```python
from build123d import *
from build123d.topology import SkipClean

# Parameters (mm, degrees)
SKETCH2_R            = 1.55
SKETCH2_R_2          = 15.6
BOSS_EXTRUDE1_DEPTH  = 5
BOSS_EXTRUDE3_DEPTH  = 41
BOSS_EXTRUDE4_DEPTH  = 7.5
BOSS_EXTRUDE5_DEPTH  = 3
BOSS_EXTRUDE6_START  = -7.5
BOSS_EXTRUDE6_DEPTH  = 10.5
SKETCH12_W           = 10.5
SKETCH12_H           = 5
BOSS_EXTRUDE8_DEPTH  = 23.65
SKETCH13_W           = 10.5
SKETCH13_H           = 5
BOSS_EXTRUDE9_DEPTH  = 23.65
SKETCH14_W           = 5
SKETCH14_H           = 28.65
CUT_EXTRUDE1_DEPTH   = 41
SKETCH15_W           = 5
SKETCH15_H           = 10.5
BOSS_EXTRUDE10_DEPTH = 13.449158782
BOSS_EXTRUDE11_DEPTH = 5
BOSS_EXTRUDE12_DEPTH = 5


# Read off the part's stored shape, not the designer's step: Boss-Extrude6
with BuildPart() as part:
    # Sketch2 → Boss-Extrude1 (new body)
    with BuildSketch(Plane.XY):
        Polygon((-10.909227683, 21.454823411), (23.390772317, 21.454823411), (27.390772317, 17.454823411), (27.390772317, -16.845176589), (23.390772317, -20.845176589), (-10.909227683, -20.845176589), (-14.909227683, -16.845176589), (-14.909227683, 17.454823411), align=None)
        with Locations((-9.359227683, 15.904823411)):
            Circle(SKETCH2_R, mode=Mode.SUBTRACT)
        with Locations(Location((21.840772317, 15.904823411, 0), (0, 0, 180))):
            Circle(SKETCH2_R, mode=Mode.SUBTRACT)
        with Locations((21.840772317, -15.295176589)):
            Circle(SKETCH2_R, mode=Mode.SUBTRACT)
        with Locations(Location((-9.359227683, -15.295176589, 0), (0, 0, 180))):
            Circle(SKETCH2_R, mode=Mode.SUBTRACT)
        with Locations((6.240772317, 0.304823411)):
            Circle(SKETCH2_R_2, mode=Mode.SUBTRACT)
    extrude(amount=BOSS_EXTRUDE1_DEPTH)

    # Sketch4 → Boss-Extrude3 (add)
    with BuildSketch(Plane.XY.offset(5)):
        Polygon((-14.909227683, -12.195176589), (-14.909227683, 0.304823411), (-14.909227683, 12.804823411), (-19.909227683, 12.804823411), (-19.909227683, -12.195176589), (-19.909227683, -20.951034478), (-10.909227683, -20.845176589), (-14.909227683, -16.845176589), align=None)
        Polygon((32.390772317, 12.804823411), (27.390772317, 12.804823411), (27.390772317, 0.304823411), (27.390772317, -12.195176589), (27.390772317, -16.845176589), (23.390772317, -20.845176589), (32.390772317, -21.056892366), (32.390772317, -12.195176589), align=None)
    extrude(amount=-BOSS_EXTRUDE3_DEPTH)

    # Sketch12 → Boss-Extrude8 (add)
    with BuildSketch(Plane.ZY.offset(-3.740772317)):
        with Locations((-41.25, -18.345176589)):
            Rectangle(SKETCH12_W, SKETCH12_H)
    extrude(amount=BOSS_EXTRUDE8_DEPTH)

    # Sketch13 → Boss-Extrude9 (add)
    with BuildSketch(Plane(origin=(8.740772317, 0, 0), x_dir=(0, 0, -1), z_dir=(1, 0, 0))):
        with Locations((41.25, -18.345176589)):
            Rectangle(SKETCH13_W, SKETCH13_H)
    extrude(amount=BOSS_EXTRUDE9_DEPTH)

    # Sketch14 → Cut-Extrude1 (cut)
    with BuildSketch(Plane(origin=(0, 0, -36), x_dir=(-1, 0, 0), z_dir=(0, 0, -1))):
        with Locations((-29.890772317, -1.520176589)):
            Rectangle(SKETCH14_W, SKETCH14_H)
        with Locations((17.409227683, -1.520176589)):
            Rectangle(SKETCH14_W, SKETCH14_H)
    extrude(amount=-CUT_EXTRUDE1_DEPTH, mode=Mode.SUBTRACT)



with BuildPart() as body_2:
    # Sketch5 → Boss-Extrude4 (new body)
    with BuildSketch(Plane(origin=(0, 0, -36), x_dir=(-1, 0, 0), z_dir=(0, 0, -1))):
        with BuildLine():
            ThreePointArc((1.459227683, 4.190775675), (-6.240772317, -8.320176589), (-13.940772317, 4.190775675))
            Line((-13.940772317, 4.190775675), (-13.940772317, 11.190775675))
            Line((-13.940772317, 11.190775675), (-13.940772317, 14.190775675))
            Line((-13.940772317, 14.190775675), (-16.940772317, 14.190775675))
            Line((-16.940772317, 14.190775675), (-16.940772317, 4.849119286))
            ThreePointArc((-16.940772317, 4.849119286), (-6.240772317, -11.320176589), (4.459227683, 4.849119286))
            Line((4.459227683, 4.849119286), (4.459227683, 14.190775675))
            Line((4.459227683, 14.190775675), (1.459227683, 14.190775675))
            Line((1.459227683, 14.190775675), (1.459227683, 11.190775675))
            Line((1.459227683, 11.190775675), (1.459227683, 4.190775675))
        make_face()
    extrude(amount=BOSS_EXTRUDE4_DEPTH)

    # Sketch6 → Boss-Extrude5 (add)
    with SkipClean():  # the faces are left unmerged after this step: merging them gives an invalid solid
        with BuildSketch(Plane(origin=(0, 0, -43.5), x_dir=(-1, 0, 0), z_dir=(0, 0, -1))):
            with BuildLine():
                Line((-16.940772317, 4.849119286), (-16.940772317, 14.190775675))
                Line((-16.940772317, 14.190775675), (4.459227683, 14.190775675))
                Line((4.459227683, 14.190775675), (4.459227683, 4.849119286))
                ThreePointArc((4.459227683, 4.849119286), (-6.240772317, -11.320176589), (-16.940772317, 4.849119286))
            make_face()
        extrude(amount=BOSS_EXTRUDE5_DEPTH)

    # Boss-Extrude6 outline → Boss-Extrude6 (add)
    with SkipClean():  # the faces are left unmerged after this step: merging them gives an invalid solid
        with BuildSketch(Plane(origin=(0, 0, -43.5), x_dir=(-1, 0, 0), z_dir=(0, 0, -1)).offset(BOSS_EXTRUDE6_START)):
            with BuildLine():
                Line((-8.740772317, -20.845176589), (-3.740772317, -20.845176589))
                Line((-3.740772317, -20.845176589), (-3.740772317, -11.048177294))
                ThreePointArc((-3.740772317, -11.048177294), (-6.240772317, -11.320176589), (-8.740772317, -11.048177294))
                Line((-8.740772317, -11.048177294), (-8.740772317, -20.845176589))
            make_face()
            with BuildLine():
                Line((-32.390772317, -2.396017807), (-17.547676478, -2.396017807))
                ThreePointArc((-17.547676478, -2.396017807), (-17.863953086, 0.099168806), (-17.636143917, 2.603982193))
                Line((-17.636143917, 2.603982193), (-32.390772317, 2.603982193))
                Line((-32.390772317, 2.603982193), (-32.390772317, -2.396017807))
            make_face()
            with BuildLine():
                ThreePointArc((5.154599283, 2.603982193), (5.382408452, 0.099168806), (5.066131844, -2.396017807))
                Line((5.066131844, -2.396017807), (19.909227683, -2.396017807))
                Line((19.909227683, -2.396017807), (19.909227683, 2.603982193))
                Line((19.909227683, 2.603982193), (5.154599283, 2.603982193))
            make_face()
        extrude(amount=BOSS_EXTRUDE6_DEPTH)


with BuildPart() as part_1:
    with SkipClean():  # the faces are left unmerged after this step: merging them gives an invalid solid
        add(part.part)

        add(body_2.part)  # Boss-Extrude10 merges body 2
        # Sketch15 → Boss-Extrude10 (add)
        with BuildSketch(Plane(origin=(0, -15.845176589, 0), x_dir=(1, 0, 0), z_dir=(0, 1, 0))):
            with Locations((29.890772317, 41.25)):
                Rectangle(SKETCH15_W, SKETCH15_H)
            with Locations((-17.409227683, 41.25)):
                Rectangle(SKETCH15_W, SKETCH15_H)
        extrude(amount=BOSS_EXTRUDE10_DEPTH)

    # Sketch16 → Boss-Extrude11 (add)
    with SkipClean():  # the faces are left unmerged after this step: merging them gives an invalid solid
        with BuildSketch(Plane(origin=(32.390772317, 0, 0), x_dir=(0, 0, -1), z_dir=(1, 0, 0))):
            Polygon((36, -10.845176589), (31, -15.845176589), (36, -15.845176589), align=None)
        extrude(amount=-BOSS_EXTRUDE11_DEPTH)

    # Sketch18 → Boss-Extrude12 (add)
    with SkipClean():  # the faces are left unmerged after this step: merging them gives an invalid solid
        with BuildSketch(Plane.ZY.offset(19.909227683)):
            Polygon((-36, -10.845176589), (-31, -15.845176589), (-36, -15.845176589), align=None)
        extrude(amount=-BOSS_EXTRUDE12_DEPTH)


solid = part_1.part
```
Verification items for the finished model (mm, model axes). A direction names the side the tool comes from. Give positions to 0.01 mm unless a question says otherwise; leave off trailing zeros. Order: outer loops, then holes, each group sorted by start corner. A loop starts at its lowest first (then second) coordinate and runs counter-clockwise, first axis right, second up. Notation, with made-up numbers: (55, 86.5) - (74, 86.5) arc R15 cw to (74, 109.5) - close; hole circle Ø7 at (11, -38.75). An arc over 180 degrees is marked (long way). Answer as CSV lines item,"result". Start each with the question number.
Item 1: Section check C-C, the plane z = -42. Record the boundary of the cut face in (x, y) (3 decimals), plus the area to 3 significant figures.
Item 2: Section check A-A, the plane z = -3. Record the boundary of the cut face in (x, y).
Item 3: Section check D-D, the plane y = -6. Record the boundary of the cut face in (x, z).
Item 4: Gauge pin test, flat ends, axial feed: pin 1 (6 mm diameter, centred on y = 10.5, z = -39.5, fed in from +X); pin 2 (3 mm diameter, centred on x = -10, z = -39, fed in from -Y); pin 3 (10 mm diameter, centred on y = -11.5, z = -32.5, fed in from +X); pin 4 (6 mm diameter, centred on y = 7.5, z = -39, fed in from -X). Record the tip position at first contact, or that the pin passes through.
Item 5: Mould release check, pull along X, two halves, no side actions. Record for faces 1 (the face through (29.926, -13.31, -33.535)), 2 (the face through (27.391, 1, 2)), 3 (the face through (6, -20.845, 2)): released by +X, released by -X, zero draft, split by the parting line, or undercut.
Item 6: Material ranges on L1, parallel to X at y = -13, z = -42.5; L2, parallel to Z at x = 11, y = 4; L3, parallel to Y at x = 28.5, z = -17, recorded low to high.
Item 7: Access from +Z, -Z, +X, -X, +Y, -Y to the whole of each face (thin tool, end or side, straight path). Record for faces 4 (the face through (-3, 15, 0)), 5 (the face through (-10, -2.396, -41)), 6 (the face through (22.674, -13.988, 2.465)).
Filled in:
1,outline,"(-19.909, -20.845) - (32.391, -20.845) - (32.391, 2.604) - (17.636, 2.604) arc R11.625 ccw to (16.941, 4.849) - (16.941, 14.191) - (13.941, 14.191) - (13.941, 4.191) arc R8.625 cw (long way) to (-1.459, 4.191) - (-1.459, 14.191) - (-4.459, 14.191) - (-4.459, 4.849) arc R11.625 ccw to (-5.155, 2.604) - (-19.909, 2.604) - close; hole (-14.909, -15.845) - (3.741, -15.845) - (3.741, -11.048) arc R11.625 cw to (-5.066, -2.396) - (-14.909, -2.396) - close; hole (8.741, -15.845) - (27.391, -15.845) - (27.391, -2.396) - (17.548, -2.396) arc R11.625 cw to (8.741, -11.048) - close"
1,area,"745 mm^2"
2,outline,"(-19.91, -20.95) - (-10.91, -20.85) - (-14.91, -16.85) - (-14.91, -15.85) - (-19.91, -15.85) - close; (23.39, -20.85) - (32.39, -21.06) - (32.39, -15.85) - (27.39, -15.85) - (27.39, -16.85) - close"
3,outline,"(-19.91, -46.5) - (-14.91, -46.5) - (-14.91, -36) - (-19.91, -36) - close; (-14.91, 0) - (-8.03, 0) - (-8.03, 5) - (-14.91, 5) - close; (-3.53, -46.5) - (16.01, -46.5) - (16.01, -36) - (12.13, -36) - (12.13, -43.5) - (0.36, -43.5) - (0.36, -36) - (-3.53, -36) - close; (20.51, 0) - (27.39, 0) - (27.39, 5) - (20.51, 5) - close; (27.39, -46.5) - (32.39, -46.5) - (32.39, -36) - (27.39, -36) - close"
4,pin 1,"x = 16.94"
4,pin 2,"y = -20.85"
4,pin 3,"x = 32.39"
4,pin 4,"x = -4.6"
5,face 1,"zero draft"
5,face 2,"released by +X"
5,face 3,"undercut"
6,L1,"-19.91 to -14.91, 3.74 to 8.74, 27.39 to 32.39"
6,L2,"-46.5 to -43.5"
6,L3,"-20.97 to -15.85"
7,face 4,"+Y"
7,face 5,"-Z"
7,face 6,"+Z"
